```python
from build123d import *

# Parameters (mm, degrees)
F0_W     = 45
F0_H     = 62.5
F1_DEPTH = 8
F3_D     = 9
F3_DEPTH = 15
F3_TIP   = 2.7038727856
F5_DEPTH = 45


with BuildPart() as f1:
    # F0 (on Top) → F1 (new body)
    with BuildSketch(Plane.XY):
        with Locations((22.5, -31.25)):
            Rectangle(F0_W, F0_H)
    extrude(amount=F1_DEPTH)

    # F3
    with Locations(Plane.XY.offset(8)):
        with Locations((12.5, -16.25), (32.5, -16.25), (32.5, -46.25), (12.5, -46.25)):
            Hole(F3_D / 2, depth=F3_DEPTH)
            with Locations((0, 0, -(F3_DEPTH + F3_TIP / 2))):  # 118° drill point
                Cone(0, F3_D / 2, F3_TIP, mode=Mode.SUBTRACT)

    # F4 (on face) → F5 (join)
    with BuildSketch(Plane.YZ.offset(45)):
        with BuildLine():
            ThreePointArc((-62.5, 1.3074175964), (-62.1260593981, 2.6306936062), (-62, 4))
            ThreePointArc((-62, 4), (-62.1260593981, 5.3693063938), (-62.5, 6.6925824036))
            Line((-62.5, 6.6925824036), (-62.5, 1.3074175964))
        make_face()
        with BuildLine():
            Line((-62.5, 1.3074175964), (-62.5, 6.6925824036))
            ThreePointArc((-62.5, 6.6925824036), (-77, 4), (-62.5, 1.3074175964))
        make_face()
        with BuildLine():
            ThreePointArc((14.5, 4), (8.3693063938, 11.3739406019), (0, 6.6925824036))
            Line((0, 6.6925824036), (0, 1.3074175964))
            ThreePointArc((0, 1.3074175964), (8.3693063938, -3.3739406019), (14.5, 4))
        make_face()
    extrude(amount=-F5_DEPTH)


solid = f1.part
```
CAD build for the part. Positions are in the model's coordinates, mm. A direction names the side the tool comes from. Round coordinates to 2 decimals unless told otherwise and drop trailing zeros. Write each loop counter-clockwise with the first axis right and the second up, starting at its lowest first coordinate (ties: lowest second). Pieces come first, ordered by that corner, then holes. Notation, with made-up numbers: (20.25, 26) -> (67.25, 26) arc R12 cw to (67.25, 41) -> close; hole circle Ø7 at (41.5, 54). An arc over 180 degrees is marked (long way). Answer in a Markdown table with one row per item. Add a question column.
Item 1: Which spindle directions (+Z, -Z, +X, -X, +Y, -Y) get a long thin tool onto all of the face, cutting with end or side? Do faces 1 (the face through (10.42, -50.24, 3.94)), 2 (the face through (22, -31, 8)). Say none if no direction does.
Item 2: Saw through at B-B, the plane x = 12.5. Write the cut outline in (y, z).
Item 3: Saw through at C-C, the plane z = -2.5. Write the cut outline in (x, y), then the cut area to 4 significant figures.
Item 4: Drop flat-ended pins along their axis: pin 1 Ø6 at (x, y) = (33, -29.5) entering from -Z; pin 2 Ø1.4 at (x, z) = (24.5, 1) entering from -Y; pin 3 Ø1.5 at (x, z) = (13, 0.5) entering from +Y; pin 4 Ø5.5 at (x, y) = (32.5, -16.25) entering from +Z. Give the stop position or say it passes through.
Item 5: Saw through at A-A, the plane y = -16.25. Write the cut outline in (x, z).
Item 6: Mould opens along Y. For faces 3 (the face through (22, -31, 0)), 4 (the face through (0, -32, 4)) say: pulls with the +Y half, pulls with the -Y half, needs draft (parallel to the pull), parting line crosses it, or undercut.
Item 7: Drill centre lines: line 1 (Y direction, x = 32.5, z = 4.5); line 2 (Y direction, x = 16.5, z = 4.5); line 3 (Z direction, x = 38.5, y = -17.5). Where is each one in solid material? Low to high. Write a range as from..to.
Item 8: Saw through at D-D, the plane x = 26. Write the cut outline in (y, z).
Findings below:
| question | item | result |
|---|---|---|
| 1 | face 1 | +Z, -Z |
| 1 | face 2 | +Z, +X, -X |
| 2 | outline | (-62.5, 0) -> (-50.75, 0) -> (-50.75, 8) -> (-62.5, 8) -> (-62.5, 6.69) arc R7.5 ccw (long way) to (-62.5, 1.31) -> close; (-41.75, 0) -> (-20.75, 0) -> (-20.75, 8) -> (-41.75, 8) -> close; (-11.75, 0) -> (0, 0) -> (0, 1.31) arc R7.5 ccw (long way) to (0, 6.69) -> (0, 8) -> (-11.75, 8) -> close |
| 3 | outline | (0, -73.24) -> (45, -73.24) -> (45, -65.76) -> (0, -65.76) -> close; (0, 3.26) -> (45, 3.26) -> (45, 10.74) -> (0, 10.74) -> close |
| 3 | area | 673.5 mm^2 |
| 4 | pin 1 | stops at z = 0 |
| 4 | pin 2 | stops at y = -76.64 |
| 4 | pin 3 | stops at y = 13.98 |
| 4 | pin 4 | passes through |
| 5 | outline | (0, 0) -> (8, 0) -> (8, 8) -> (0, 8) -> close; (17, 0) -> (28, 0) -> (28, 8) -> (17, 8) -> close; (37, 0) -> (45, 0) -> (45, 8) -> (37, 8) -> close |
| 6 | face 3 | undercut |
| 6 | face 4 | needs draft |
| 7 | line 1 | y = -76.98..-50.75, -41.75..-20.75, -11.75..14.48 |
| 7 | line 2 | y = -76.98..-48.31, -44.19..-18.31, -14.19..14.48 |
| 7 | line 3 | z = 0..8 |
| 8 | outline | (-62.5, 0) -> (0, 0) -> (0, 1.31) arc R7.5 ccw (long way) to (0, 6.69) -> (0, 8) -> (-62.5, 8) -> (-62.5, 6.69) arc R7.5 ccw (long way) to (-62.5, 1.31) -> close |
